Input: part model. Units: mm. Frame: model coordinates. Face numbers are marked on the shaded views. Coordinates: 2 decimals unless noted, no trailing zeros. Order: outer loops, then holes, each group sorted by start corner. A loop starts at its lowest first (then second) coordinate and runs counter-clockwise, first axis right, second up. Notation, with made-up numbers: (64, -15.5) -> (75, -15.5) arc R19 ccw to (75, 13.5) -> close; hole circle Ø8 at (-2.75, -23). An arc over 180 degrees is marked (long way). One line per item, written item: value. Start each with the question number.
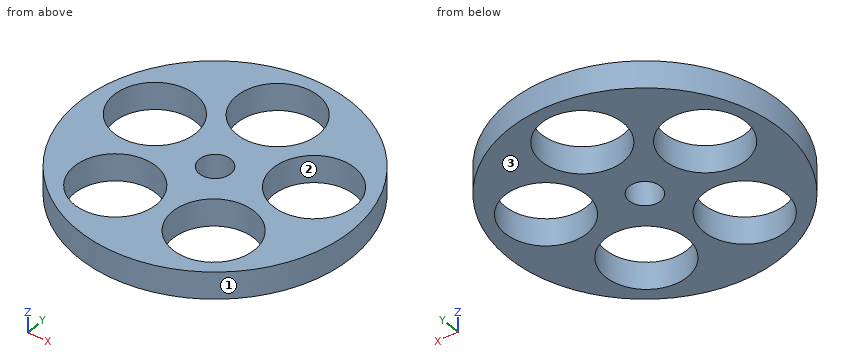
Autodesk Fusion 360 part; units mm, degrees
sketch "Sketch1" plane through (0, 0, 0) normal (0, 0, 1) x (1, 0, 0)
  circle A0 centre (0, 0) radius 1.15
  circle A1 centre (0, 0) radius 10
  circle A2 centre (0.008, 6.0716) radius 3
  circle A3 centre (-5.772, 1.8838) radius 3
  circle A4 centre (-3.5753, -4.9074) radius 3
  circle A5 centre (3.5623, -4.9168) radius 3
  circle A6 centre (5.7769, 1.8686) radius 3
  dimension "d1" = 2.3
  dimension "d2" = 20
  dimension "d3" = 6
  dimension "d5" = 360
extrude "Extrude1" add sketch "Sketch1" along normal blind 2
1) Mould query, pull axis X, two halves, no side actions, for the marked faces 1, 2 and 3. Classes: +X half, -X half, draft (parallel to the pull), parting line (faces both ways), or undercut.
2) Section query D-D, the plane z = 0.35. Return the cut outline in (x, y).
3) Ray query, line 1 along Y through (x, z) = (-0.25, 1.7); line 2 along X through (y, z) = (2.5, 1.6); line 3 along Y through (x, z) = (6, 1.95). Return the intervals inside material, ascending. Write a range as from..to.
4) Section query B-B, the plane y = 5.75. Return the cut outline in (x, z), plus the area to 3 significant figures.
5) Pin query (flat end, axial travel): pin 1 Ø1 at (x, y) = (7, -4) entering from -Z. Return the tip coordinate at first contact, or that it passes through.
6) Section query C-C, the plane x = 3.5. Return the cut outline in (y, z), plus the area to 3 significant figures.
7) Section query A-A, the plane y = -6.75. Return the cut outline in (x, z), plus the area to 3 significant figures.
Entries:
1. face 1: parting line
1. face 2: undercut
1. face 3: draft
2. outline: circle Ø20 at (0, 0); hole circle Ø6 at (-5.77, 1.88); hole circle Ø6 at (-3.58, -4.91); hole circle Ø6 at (0.01, 6.07); hole circle Ø2.3 at (0, 0); hole circle Ø6 at (3.56, -4.92); hole circle Ø6 at (5.78, 1.87)
3. line 1: y = -10..-1.12, 1.12..3.08, 9.06..10
3. line 2: x = -9.68..-8.71, -2.84..2.84, 8.71..9.68
3. line 3: y = -8..-6.67, -3.17..-1.12, 4.86..8
4. outline: (-8.18, 0) -> (-2.97, 0) -> (-2.97, 2) -> (-8.18, 2) -> close; (2.99, 0) -> (8.18, 0) -> (8.18, 2) -> (2.99, 2) -> close
4. area: 20.8 mm2
5. pin 1: stops at z = 0
6. outline: (-9.37, 0) -> (-7.92, 0) -> (-7.92, 2) -> (-9.37, 2) -> close; (-1.92, 0) -> (-0.08, 0) -> (-0.08, 2) -> (-1.92, 2) -> close; (3.82, 0) -> (9.37, 0) -> (9.37, 2) -> (3.82, 2) -> close
6. area: 17.7 mm2
7. outline: (-7.38, 0) -> (-5.94, 0) -> (-5.94, 2) -> (-7.38, 2) -> close; (-1.21, 0) -> (1.19, 0) -> (1.19, 2) -> (-1.21, 2) -> close; (5.94, 0) -> (7.38, 0) -> (7.38, 2) -> (5.94, 2) -> close
7. area: 10.5 mm2
